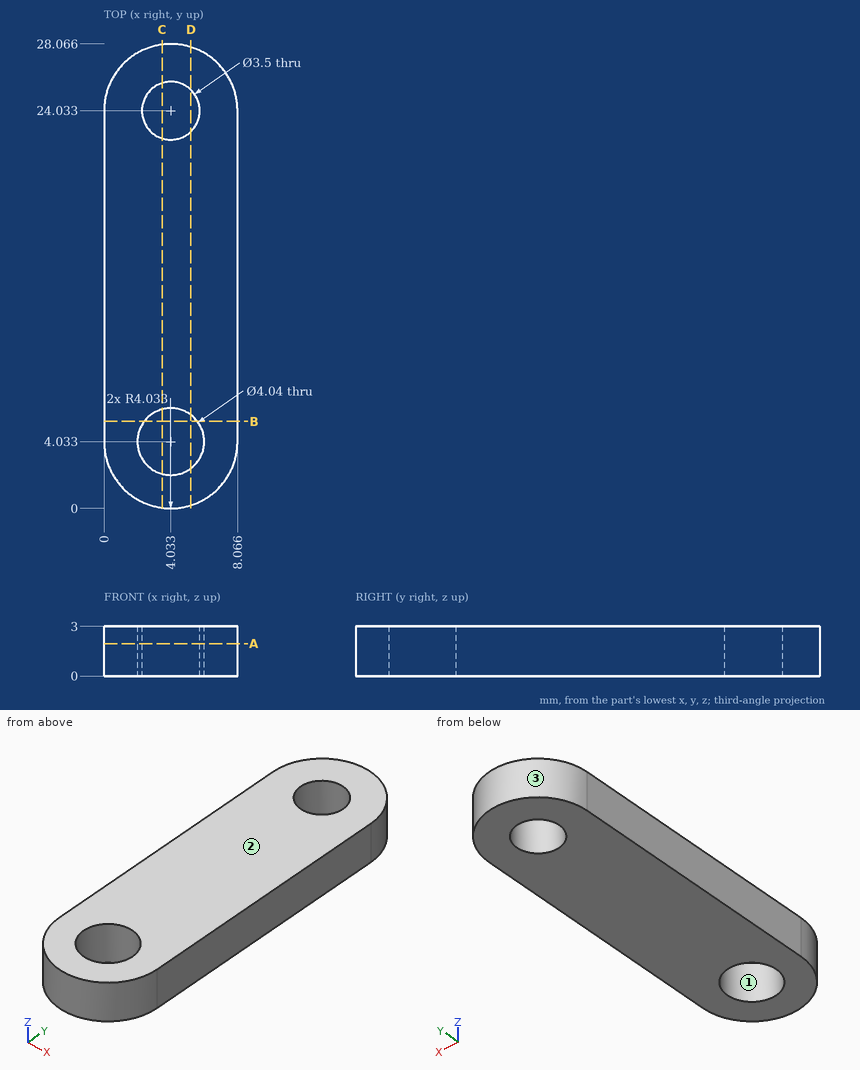
For this review, use the dimensioned drawing (mm, ordinates from the lowest corner) and the shaded views. Give positions to 0.01 mm unless a question says otherwise; leave off trailing zeros. Write each loop counter-clockwise with the first axis right and the second up, starting at its lowest first coordinate (ties: lowest second). Pieces come first, ordered by that corner, then holes. Notation, with made-up numbers: M 78.5,65.25 L 137.5,65.25 A15 ccw 137.5,78.25 Z; hole C -27,-21.75 d6. An arc over 180 degrees is marked long. Answer as a JSON object with one key per item and string values. Group by question number.
1) For line 1 along Y through (x, z) = (5.5, 0.35) (1 decimal); line 2 along X through (y, z) = (24, 2.4); line 3 along X through (y, z) = (4.25, 2.15) (1 decimal), list the stretches that pass through material, from the lowest coordinate up.
2) We need section B-B (y = 5.25). Give the boundary of the cut face in (x, z) (1 decimal), and give its area (3 significant figures).
3) We need section C-C (x = 3.5). Give the boundary of the cut face in (y, z) (1 decimal), and give its area (3 significant figures).
4) We need section A-A (z = 1.95). Give the boundary of the cut face in (x, y).
5) Clearance check with a flat-ended pin moving along its axis: pin 1 Ø1 at (x, z) = (6.5, 1.5) entering from -Y. State where the tip first meets the part, or that it passes through.
6) We need section D-D (x = 5.25). Give the boundary of the cut face in (y, z) (1 decimal).
7) Mouldability with a two-part tool opening along Y and no side actions: class the marked faces 1, 2 and 3 as released by +Y, released by -Y, zero draft, split by the parting line, or undercut.
Answer key:
{
 "1": {"line 1": "y = 0.3 to 2.6, 5.4 to 23.1, 25 to 27.8", "line 2": "x = 0 to 2.28, 5.78 to 8.07", "line 3": "x = 0 to 2, 6 to 8.1"},
 "2": {"outline": "M 0,0 L 2.4,0 L 2.4,3 L 0,3 Z; M 5.6,0 L 8.1,0 L 8.1,3 L 5.6,3 Z", "area": "14.5 mm²"},
 "3": {"outline": "M 0,0 L 2.1,0 L 2.1,3 L 0,3 Z; M 6,0 L 22.4,0 L 22.4,3 L 6,3 Z; M 25.7,0 L 28,0 L 28,3 L 25.7,3 Z", "area": "62.3 mm²"},
 "4": {"outline": "M 0,4.03 A4.03 ccw 8.07,4.03 L 8.07,24.03 A4.03 ccw 0,24.03 Z; hole C 4.03,4.03 d4.04; hole C 4.03,24.03 d3.5"},
 "5": {"pin 1": "stops at y = 0.51"},
 "6": {"outline": "M 0.2,0 L 2.4,0 L 2.4,3 L 0.2,3 Z; M 5.6,0 L 22.8,0 L 22.8,3 L 5.6,3 Z; M 25.3,0 L 27.9,0 L 27.9,3 L 25.3,3 Z"},
 "7": {"face 1": "undercut", "face 2": "zero draft", "face 3": "released by +Y"}
}
